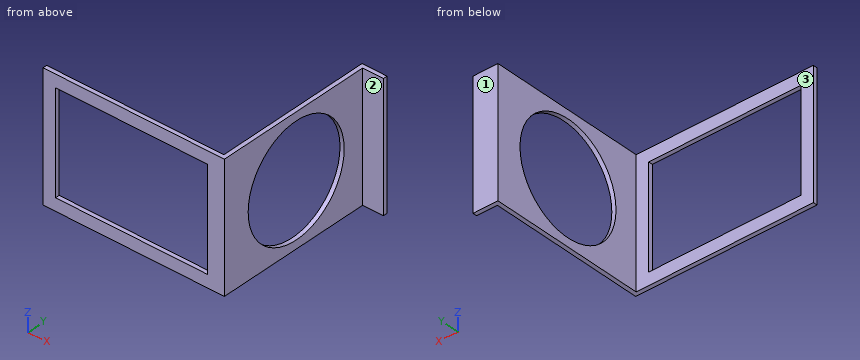
from build123d import *

# Parameters (mm, degrees)
F0_W     = 213
F0_H     = 152
F0_W_2   = 183
F0_H_2   = 122
F1_DEPTH = 5
F2_W     = 185
F2_H     = 152
F2_W_2   = 5
F3_DEPTH = 5
F4_R     = 66
F5_DEPTH = 25
F6_W     = 25
F6_H     = 152
F6_W_2   = 5
F7_DEPTH = 5


with BuildPart() as f1:
    # F0 (on Front) → F1 (new body)
    with BuildSketch(Plane.XZ):
        with Locations((-0.431097, 6.392034)):
            Rectangle(F0_W, F0_H)
        with Locations((-0.431097, 6.392034)):
            Rectangle(F0_W_2, F0_H_2, mode=Mode.SUBTRACT)
    extrude(amount=F1_DEPTH)

    # F2 (on face) → F3 (join)
    with BuildSketch(Plane.YZ.offset(106.068903)):
        with Locations((92.5, 6.392034)):
            Rectangle(F2_W, F2_H)
        with Locations((-2.5, 6.392034)):
            Rectangle(F2_W_2, F2_H)
    extrude(amount=F3_DEPTH)

    # F4 (on face) → F5 (cut)
    with BuildSketch(Plane.YZ.offset(111.068903)):
        with Locations((93.713939, 6.392034)):
            Circle(F4_R)
    extrude(amount=-F5_DEPTH, mode=Mode.SUBTRACT)

    # F6 (on face) → F7 (join)
    with BuildSketch(Plane(origin=(0, 185, 0), x_dir=(-1, 0, 0), z_dir=(0, 1, 0))):
        with Locations((-123.568903, 6.392034)):
            Rectangle(F6_W, F6_H)
        with Locations((-108.568903, 6.392034)):
            Rectangle(F6_W_2, F6_H)
    extrude(amount=F7_DEPTH)


solid = f1.part
Build history of the part. All positions in model axes, mm. Face numbers are marked on the shaded views. A direction names the side the tool comes from. Round coordinates to 2 decimals unless told otherwise and drop trailing zeros. Write each loop counter-clockwise with the first axis right and the second up, starting at its lowest first coordinate (ties: lowest second). Pieces come first, ordered by that corner, then holes. Notation, with made-up numbers: (37, -19) -> (50, -19) arc R23 cw to (50, 4) -> close; hole circle Ø4 at (33, 19.5). An arc over 180 degrees is marked (long way). Write item = value, one per line.
(1) Band-saw the part on C-C (y = 97). Give the cut face in (x, z).
Answer:
outline = (106.07, -69.61) -> (111.07, -69.61) -> (111.07, -59.53) -> (106.07, -59.53) -> close; (106.07, 72.31) -> (111.07, 72.31) -> (111.07, 82.39) -> (106.07, 82.39) -> close
(2) Band-saw the part on B-B (z = -47.5). Give the cut face in (x, y), then the cut area to 3 significant figures.
Answer:
outline = (-106.93, -5) -> (-91.93, -5) -> (-91.93, 0) -> (-106.93, 0) -> close; (91.07, -5) -> (111.07, -5) -> (111.07, 55.61) -> (106.07, 55.61) -> (106.07, 0) -> (91.07, 0) -> close; (106.07, 131.81) -> (111.07, 131.81) -> (111.07, 185) -> (136.07, 185) -> (136.07, 190) -> (106.07, 190) -> close
area = 869 mm2
(3) Probe L1, parallel to X at y = 20, z = -37; L2, parallel to Y at x = 43.5, z = -62; L3, parallel to Y at x = 114, z = 19.5. List the from-to ranges inside material, lowest first.
Answer:
L1 = 106.07 to 111.07
L2 = -5 to 0
L3 = 185 to 190
(4) Band-saw the part on A-A (x = -1.5). Give the cut face in (y, z), then the cut area to 3 significant figures.
Answer:
outline = (-5, -69.61) -> (0, -69.61) -> (0, -54.61) -> (-5, -54.61) -> close; (-5, 67.39) -> (0, 67.39) -> (0, 82.39) -> (-5, 82.39) -> close
area = 150 mm2
(5) Band-saw the part on D-D (z = -0.5). Give the cut face in (x, y), then the cut area to 3 significant figures.
Answer:
outline = (-106.93, -5) -> (-91.93, -5) -> (-91.93, 0) -> (-106.93, 0) -> close; (91.07, -5) -> (111.07, -5) -> (111.07, 28.07) -> (106.07, 28.07) -> (106.07, 0) -> (91.07, 0) -> close; (106.07, 159.35) -> (111.07, 159.35) -> (111.07, 185) -> (136.07, 185) -> (136.07, 190) -> (106.07, 190) -> close
area = 594 mm2
(6) Tool access for the marked faces 1, 2 and 3: list every direction of +Z, -Z, +X, -X, +Y, -Y with a clear straight run to the whole face (end or side of a thin tool).
Answer:
face_1 = +Z, -Z, +X, -X, +Y
face_2 = +Z, -Z, +X, -Y
face_3 = +Z, -Z, -X, +Y
(7) Flat gauge pins, fed straight in: pin 1 (1.5 mm diameter, centred on y = -3.5, z = 24, fed in from +X); pin 2 (5 mm diameter, centred on y = 26.5, z = 21, fed in from -X); pin 3 (20 mm diameter, centred on x = 123.5, z = 34, fed in from -Y). Where does each tip first touch, or does it go through?
Answer:
pin_1 = 111.07
pin_2 = 106.07
pin_3 = 185
